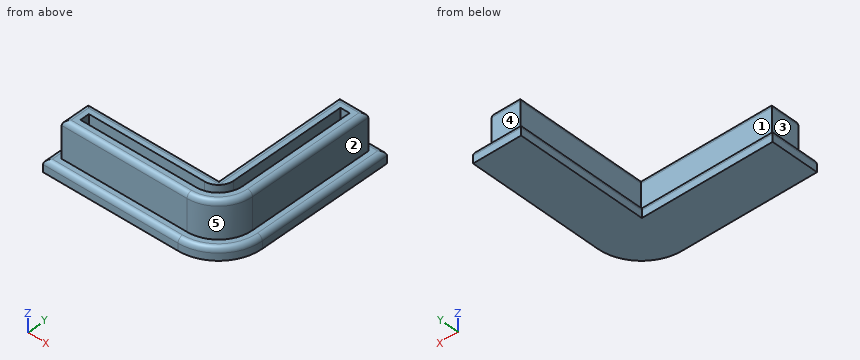
```python
from build123d import *

# Parameters (mm, degrees)
F0_W     = 2.3876
F0_H     = 2.54
F0_W_2   = 2.54
F0_H_2   = 2.3876
F1_DEPTH = 3.175
F2_DEPTH = 12.7
F3_R     = 1.27


with BuildPart() as f1:
    # F0 (on Top) → F1 (new body)
    with BuildSketch(Plane.XY):
        Polygon((-34.1249, 7.4676), (-34.1249, 4.9276), (-4.9276, 4.9276), (-4.9276, 34.1249), (-7.4676, 34.1249), (-7.4676, 7.4676), align=None)
        with Locations((-35.3187, 6.1976)):
            Rectangle(F0_W, F0_H)
        with BuildLine():
            Line((-39.0525, 4.9276), (-36.5125, 4.9276))
            Line((-36.5125, 4.9276), (-36.5125, 7.4676))
            Line((-36.5125, 7.4676), (-41.5925, 7.4676))
            Line((-41.5925, 7.4676), (-41.5925, -5.08))
            Line((-41.5925, -5.08), (-6.35, -5.08))
            ThreePointArc((-6.35, -5.08), (1.732230509, -1.732230509), (5.08, 6.35))
            Line((5.08, 6.35), (5.08, 41.5925))
            Line((5.08, 41.5925), (-7.4676, 41.5925))
            Line((-7.4676, 41.5925), (-7.4676, 36.5125))
            Line((-7.4676, 36.5125), (-4.9276, 36.5125))
            Line((-4.9276, 36.5125), (-4.9276, 39.0525))
            Line((-4.9276, 39.0525), (2.54, 39.0525))
            Line((2.54, 39.0525), (2.54, 6.35))
            ThreePointArc((2.54, 6.35), (-0.0638207153, 0.0638207153), (-6.35, -2.54))
            Line((-6.35, -2.54), (-39.0525, -2.54))
            Line((-39.0525, -2.54), (-39.0525, 4.9276))
        make_face()
        with BuildLine():
            Line((-34.1249, 4.9276), (-34.1249, 2.3876))
            Line((-34.1249, 2.3876), (-6.35, 2.3876))
            ThreePointArc((-6.35, 2.3876), (-3.5481600902, 3.5481600902), (-2.3876, 6.35))
            Line((-2.3876, 6.35), (-2.3876, 34.1249))
            Line((-2.3876, 34.1249), (-4.9276, 34.1249))
            Line((-4.9276, 34.1249), (-4.9276, 4.9276))
            Line((-4.9276, 4.9276), (-34.1249, 4.9276))
        make_face()
        with BuildLine():
            Line((-36.5125, 0), (-6.35, 0))
            ThreePointArc((-6.35, 0), (-1.8598719395, 1.8598719395), (0, 6.35))
            Line((0, 6.35), (0, 36.5125))
            Line((0, 36.5125), (-2.3876, 36.5125))
            Line((-2.3876, 36.5125), (-2.3876, 34.1249))
            Line((-2.3876, 34.1249), (-2.3876, 6.35))
            ThreePointArc((-2.3876, 6.35), (-3.5481600902, 3.5481600902), (-6.35, 2.3876))
            Line((-6.35, 2.3876), (-34.1249, 2.3876))
            Line((-34.1249, 2.3876), (-36.5125, 2.3876))
            Line((-36.5125, 2.3876), (-36.5125, 0))
        make_face()
        with BuildLine():
            ThreePointArc((0, 6.35), (-1.8598719395, 1.8598719395), (-6.35, 0))
            Line((-6.35, 0), (-36.5125, 0))
            Line((-36.5125, 0), (-36.5125, 2.3876))
            Line((-36.5125, 2.3876), (-36.5125, 4.9276))
            Line((-36.5125, 4.9276), (-39.0525, 4.9276))
            Line((-39.0525, 4.9276), (-39.0525, -2.54))
            Line((-39.0525, -2.54), (-6.35, -2.54))
            ThreePointArc((-6.35, -2.54), (-0.0638207153, 0.0638207153), (2.54, 6.35))
            Line((2.54, 6.35), (2.54, 39.0525))
            Line((2.54, 39.0525), (-4.9276, 39.0525))
            Line((-4.9276, 39.0525), (-4.9276, 36.5125))
            Line((-4.9276, 36.5125), (-2.3876, 36.5125))
            Line((-2.3876, 36.5125), (0, 36.5125))
            Line((0, 36.5125), (0, 6.35))
        make_face()
        with Locations((-35.3187, 3.6576)):
            Rectangle(F0_W, F0_H)
        with Locations((-3.6576, 35.3187)):
            Rectangle(F0_W_2, F0_H_2)
        with Locations((-6.1976, 35.3187)):
            Rectangle(F0_W_2, F0_H_2)
    extrude(amount=F1_DEPTH)

    # F0 (on Top) → F2 (join)
    with BuildSketch(Plane.XY):
        with BuildLine():
            ThreePointArc((0, 6.35), (-1.8598719395, 1.8598719395), (-6.35, 0))
            Line((-6.35, 0), (-36.5125, 0))
            Line((-36.5125, 0), (-36.5125, 2.3876))
            Line((-36.5125, 2.3876), (-36.5125, 4.9276))
            Line((-36.5125, 4.9276), (-39.0525, 4.9276))
            Line((-39.0525, 4.9276), (-39.0525, -2.54))
            Line((-39.0525, -2.54), (-6.35, -2.54))
            ThreePointArc((-6.35, -2.54), (-0.0638207153, 0.0638207153), (2.54, 6.35))
            Line((2.54, 6.35), (2.54, 39.0525))
            Line((2.54, 39.0525), (-4.9276, 39.0525))
            Line((-4.9276, 39.0525), (-4.9276, 36.5125))
            Line((-4.9276, 36.5125), (-2.3876, 36.5125))
            Line((-2.3876, 36.5125), (0, 36.5125))
            Line((0, 36.5125), (0, 6.35))
        make_face()
        with BuildLine():
            Line((-34.1249, 4.9276), (-34.1249, 2.3876))
            Line((-34.1249, 2.3876), (-6.35, 2.3876))
            ThreePointArc((-6.35, 2.3876), (-3.5481600902, 3.5481600902), (-2.3876, 6.35))
            Line((-2.3876, 6.35), (-2.3876, 34.1249))
            Line((-2.3876, 34.1249), (-4.9276, 34.1249))
            Line((-4.9276, 34.1249), (-4.9276, 4.9276))
            Line((-4.9276, 4.9276), (-34.1249, 4.9276))
        make_face()
        with Locations((-35.3187, 3.6576)):
            Rectangle(F0_W, F0_H)
        with Locations((-3.6576, 35.3187)):
            Rectangle(F0_W_2, F0_H_2)
    extrude(amount=F2_DEPTH)

    # F3
    f3_edges = [f1.edges().sort_by_distance(p)[0] for p in [
        (5.08, 23.97125, 3.175),
        (-1.1938, 41.5925, 3.175),
        (-7.4676, 24.53005, 3.175),
        (-24.53005, 7.4676, 3.175),
        (-41.5925, 1.1938, 3.175),
        (-4.9276, 21.99005, 12.7),
        (-1.1938, 39.0525, 12.7),
        (2.54, 22.70125, 12.7),
        (-21.99005, 4.9276, 12.7),
        (-39.0525, 1.1938, 12.7),
    ]]
    fillet(f3_edges, radius=F3_R)


solid = f1.part
```
Check sheet for the modelled part. Datum: model origin and axes. Units: mm. Face numbers are marked on the shaded views. A direction names the side the tool comes from. Round coordinates to 2 decimals unless told otherwise and drop trailing zeros. Order: outer loops, then holes, each group sorted by start corner. A loop starts at its lowest first (then second) coordinate and runs counter-clockwise, first axis right, second up. Notation, with made-up numbers: (-35.5, 53.5) -> (-27.5, 53.5) arc R34 cw to (-27.5, 86.5) -> close; hole circle Ø6 at (-9.5, 26). An arc over 180 degrees is marked (long way). Use CSV: the item, a comma, the result in double quotes.
(1) Cross-section at A-A (x = -19.5). Record the boundary of the cut face in (y, z) (3 decimals).
Worked out:
outline,"(-5.08, 0) -> (7.468, 0) -> (7.468, 1.905) arc R1.27 ccw to (6.198, 3.175) -> (4.928, 3.175) -> (4.928, 11.43) arc R1.27 ccw to (3.658, 12.7) -> (2.388, 12.7) -> (2.388, 3.175) -> (0, 3.175) -> (0, 12.7) -> (-1.27, 12.7) arc R1.27 ccw to (-2.54, 11.43) -> (-2.54, 3.175) -> (-3.81, 3.175) arc R1.27 ccw to (-5.08, 1.905) -> close"
(2) Material ranges on line 1 along X through (y, z) = (34.5, 8); line 2 along Y through (x, z) = (-13.5, 10.25); line 3 along Y through (x, z) = (-33.5, 1), recorded low to high. Write a range as from..to.
Worked out:
line 1,"-4.93..-2.39, 0..2.54"
line 2,"-2.54..0, 2.39..4.93"
line 3,"-5.08..7.47"
(3) Tool access check on the marked faces 1, 2, 3, 4 and 5. Record the directions out of +Z, -Z, +X, -X, +Y, -Y that give a thin tool (end or side, any length) a straight path to the whole face; none if there is none.
Worked out:
face 1,"+Z, -X, +Y"
face 2,"+Z, +X, +Y, -Y"
face 3,"+Z, -X, +Y, -Y"
face 4,"+Z, +X, -X, +Y"
face 5,"+Z, +X, -Y"
(4) Depth check by flat-ended pin: pin 1 (2.5 mm diameter, centred on y = 2, z = 10, fed in from +X); pin 2 (6 mm diameter, centred on y = 21, z = 10, fed in from -X); pin 3 (5 mm diameter, centred on x = -19, z = 9.5, fed in from -Y). Enter the tip coordinate at first touch or a pass-through.
Worked out:
pin 1,"x = 1.98"
pin 2,"x = -4.93"
pin 3,"y = -2.54"
(5) Cross-section at C-C (y = 19). Record the boundary of the cut face in (x, z) (3 decimals), and give its area (3 significant figures).
Worked out:
outline,"(-7.468, 0) -> (5.08, 0) -> (5.08, 1.905) arc R1.27 ccw to (3.81, 3.175) -> (2.54, 3.175) -> (2.54, 11.43) arc R1.27 ccw to (1.27, 12.7) -> (0, 12.7) -> (0, 3.175) -> (-2.388, 3.175) -> (-2.388, 12.7) -> (-3.658, 12.7) arc R1.27 ccw to (-4.928, 11.43) -> (-4.928, 3.175) -> (-6.198, 3.175) arc R1.27 ccw to (-7.468, 1.905) -> close"
area,"86.8 mm²"
(6) Cross-section at B-B (z = 8.5). Record the boundary of the cut face in (x, y), and give its area (3 significant figures).
Worked out:
outline,"(-39.05, -2.54) -> (-6.35, -2.54) arc R8.89 ccw to (2.54, 6.35) -> (2.54, 39.05) -> (-4.93, 39.05) -> (-4.93, 4.93) -> (-39.05, 4.93) -> close; hole (-36.51, 0) -> (-6.35, 0) arc R6.35 ccw to (0, 6.35) -> (0, 36.51) -> (-2.39, 36.51) -> (-2.39, 6.35) arc R3.96 cw to (-6.35, 2.39) -> (-36.51, 2.39) -> close"
area,"385 mm²"
